from build123d import *

# Parameters (mm, degrees)
SKETCH1_R           = 3
SKETCH1_R_2         = 8
BOSS_EXTRUDE1_DEPTH = 9
SKETCH2_R           = 8
BOSS_EXTRUDE2_DEPTH = 4
FILLET1_R           = 1


with BuildPart() as part:
    # Sketch1 → Boss-Extrude1 (new body)
    with BuildSketch(Plane(origin=(0, 0, 0), x_dir=(1, 0, 0), z_dir=(0, 1, 0))):
        with Locations((-8, 0)):
            Circle(SKETCH1_R)
        Circle(SKETCH1_R_2)
        with Locations((8, 0)):
            Circle(SKETCH1_R)
    extrude(amount=BOSS_EXTRUDE1_DEPTH)

    # Sketch2 → Boss-Extrude2 (add)
    with BuildSketch(Plane(origin=(0, 9, 0), x_dir=(1, 0, 0), z_dir=(0, 1, 0))):
        with Locations(Location((0, 0, 0), (0, 0, 158.38615425))):
            Circle(SKETCH2_R)
    extrude(amount=BOSS_EXTRUDE2_DEPTH)

    # Fillet1
    fillet1_edges = [part.edges().sort_by_distance(p)[0] for p in [
        (7.4375, 13, 2.946793809),
    ]]
    fillet(fillet1_edges, radius=FILLET1_R)


solid = part.part
Part model, mm, in its own coordinate system. Give positions to 0.01 mm unless a question says otherwise; leave off trailing zeros. Loops run counter-clockwise (first coordinate to the right, second up) from the corner with the lowest first, then second, coordinate; pieces in that order, holes last. Notation, with made-up numbers: (77, 8.5) -> (102, 8.5) arc R23 cw to (102, 47.5) -> close; hole circle Ø11 at (38.5, 63). An arc over 180 degrees is marked (long way). Write each question's results on one line, items separated by ' | '. Start each with the question number.
Q1. Wall check: L1, parallel to Y at x = 9, z = -0.75; L2, parallel to Z at x = -4, y = 9.25; L3, parallel to X at y = 5.5, z = -0.25. Give the ranges that are in metal, low to high.
Q2. Band-saw the part on A-A on z = 0. List the corners of the cut face in (x, y).
Q3. Pin check, flat tips, straight feed: P1, Ø5, axis at x = 5.5, z = 6, coming from the -Y side; P2, Ø1.5, axis at x = -8.5, y = 6, coming from the +Z side; P3, Ø3, axis at x = 7.5, y = 6.5, coming from the +Z side; P4, Ø5, axis at x = -5, y = 9.5, coming from the +Z side. Stop position of each tip, or through.
Q4. Band-saw the part on B-B on y = 2.5. List the corners of the cut face in (x, z).
Results are:
1) L1: y = 0 to 9 | L2: z = -6.93 to 6.93 | L3: x = -10.99 to 10.99
2) outline: (-11, 0) -> (11, 0) -> (11, 9) -> (8, 9) -> (8, 12) arc R1 ccw to (7, 13) -> (-7, 13) arc R1 ccw to (-8, 12) -> (-8, 9) -> (-11, 9) -> close
3) P1: stops at y = 0 | P2: stops at z = 3 | P3: stops at z = 5.29 | P4: stops at z = 7.6
4) outline: (-7.44, -2.95) arc R8 ccw to (7.44, -2.95) arc R3 ccw (long way) to (7.44, 2.95) arc R8 ccw to (-7.44, 2.95) arc R3 ccw (long way) to start
